Can you work these out from the drawing? Everything is in mm from the part's minimum corner. A direction names the side the tool comes from. Round coordinates to 2 decimals unless told otherwise and drop trailing zeros. Order: outer loops, then holes, each group sorted by start corner. A loop starts at its lowest first (then second) coordinate and runs counter-clockwise, first axis right, second up. Notation, with made-up numbers: (5, 75.5) - (59, 75.5) arc R14 ccw to (59, 85.5) - close; hole circle Ø8 at (-12.75, -13.5). An arc over 180 degrees is marked (long way). Answer as a JSON object with one key per item and string values.
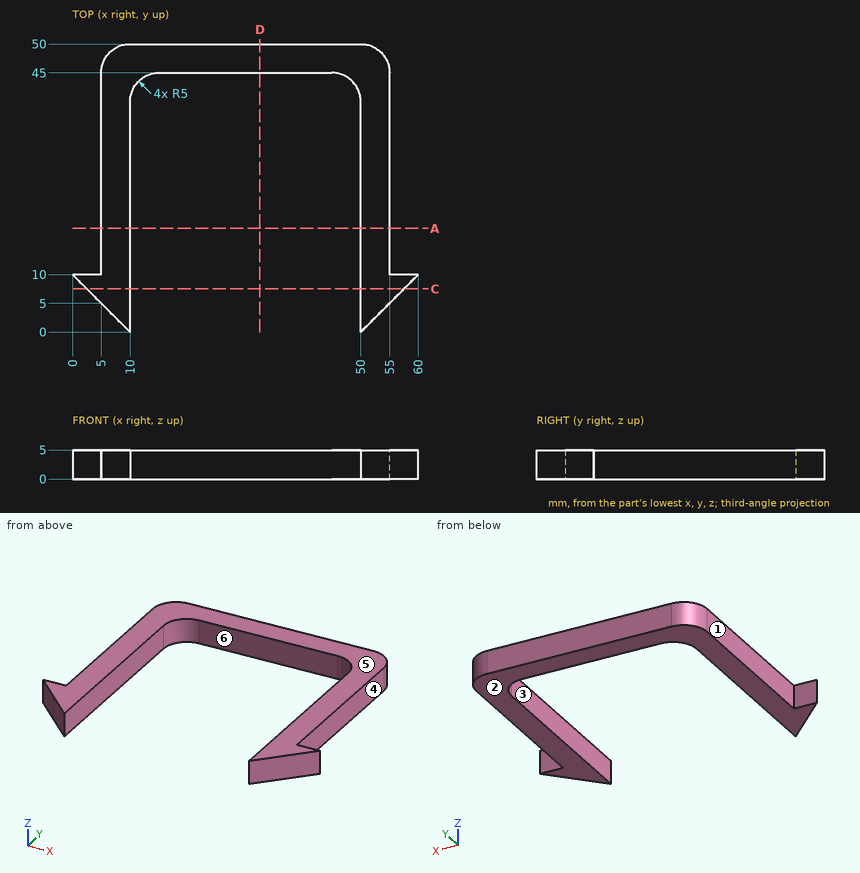
1. If I drill on L1, parallel to X at y = 29, z = 2.95; L2, parallel to X at y = 7.5, z = 2.6; L3, parallel to Y at x = 40, z = 4.45, over which ranges is the centre line in solid material (lowest first)? Write a range as [from, to].
Responses:
{"L1": "[5, 10], [50, 55]", "L2": "[2.5, 10], [50, 57.5]", "L3": "[45, 50]"}
2. Imagine slicing it at A-A (y = 18). List the corners of the cut face in (x, z) for me, plus the area to 3 significant figures.
Responses:
{"outline": "(5, 0) - (10, 0) - (10, 5) - (5, 5) - close; (50, 0) - (55, 0) - (55, 5) - (50, 5) - close", "area": "50.0 mm2"}
3. Imagine slicing it at C-C (y = 7.5). List the corners of the cut face in (x, z) for me, plus the area to 3 significant figures.
Responses:
{"outline": "(2.5, 0) - (10, 0) - (10, 5) - (2.5, 5) - close; (50, 0) - (57.5, 0) - (57.5, 5) - (50, 5) - close", "area": "75.0 mm2"}
4. Thinking about a two-plate mould opening in X: for the marked faces 4, 5 and 6, which applies, pulls with the +X half, pulls with the -X half, needs draft (parallel to the pull), parting line crosses it, or undercut?
Responses:
{"face 4": "pulls with the +X half", "face 5": "needs draft", "face 6": "undercut"}
5. For the marked faces 1, 2 and 3, which set-ups out of +Z, -Z, +X, -X, +Y, -Y let a thin tool reach every point of the face, with its end or its side?
Responses:
{"face 1": "+Z, -Z, -X, +Y", "face 2": "-Z, +X, -X, +Y, -Y", "face 3": "+Z, -Z, -Y"}
6. Imagine slicing it at D-D (x = 32.5). List the corners of the cut face in (y, z) for me, plus the area to 3 significant figures.
Responses:
{"outline": "(45, 0) - (50, 0) - (50, 5) - (45, 5) - close", "area": "25.0 mm2"}
7. For P1, Ø2.5, axis at y = 17, z = 3.5, coming from the -X side; P2, Ø2.5, axis at x = 33, z = 3, coming from the -Y side; P3, Ø2, axis at y = 36.5, z = 2.5, coming from the +X side, each with a flat end and sliding along its axis, tell me the tip position at first contact or that it passes through.
Responses:
{"P1": "x = 5", "P2": "y = 45", "P3": "x = 55"}
